The model under review builds one solid part; all positions refer to its coordinate system, in mm. Face numbers are marked on the shaded views. A direction names the side the tool comes from. Coordinates: 2 decimals unless noted, no trailing zeros. Loops run counter-clockwise (first coordinate to the right, second up) from the corner with the lowest first, then second, coordinate; pieces in that order, holes last. Notation, with made-up numbers: M 32.5,24.25 L 54.5,24.25 A14 ccw 54.5,51.25 Z; hole C 80.5,28 d5. An arc over 180 degrees is marked long. Use one line per item in the form item = value.
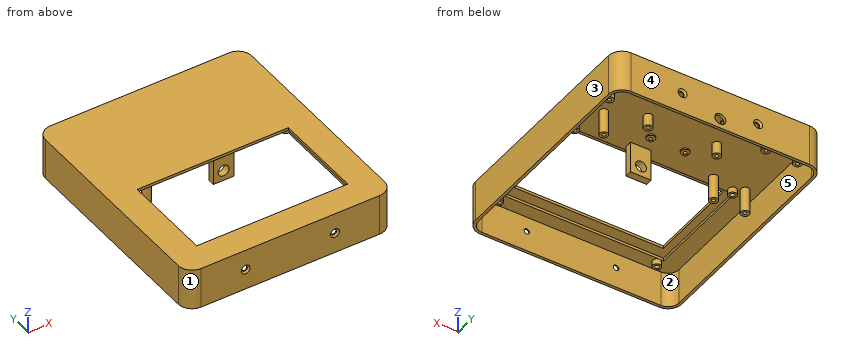
```python
from build123d import *

# Parameters (mm, degrees)
PAD_DEPTH           = 30
POCKET_DEPTH        = 26
SKETCH002_W         = 110
SKETCH002_H         = 66
POCKET001_DEPTH     = 5
SKETCH003_W         = 121
SKETCH003_H         = 78
POCKET002_DEPTH     = 2
SKETCH004_R         = 3
PAD001_DEPTH        = 4
SKETCH005_R         = 1.6
POCKET003_DEPTH     = 6
SKETCH006_R         = 3
PAD002_DEPTH        = 18
SKETCH007_R         = 1.3
POCKET004_DEPTH     = 8
SKETCH008_R         = 3
PAD003_DEPTH        = 1
SKETCH009_R         = 1
PAD004_DEPTH        = 2
SKETCH010_R         = 3
PAD005_DEPTH        = 9
SKETCH011_R         = 1.3
POCKET005_DEPTH     = 8
HOLE_D              = 4
HOLE_DEPTH          = 23.798279
HOLE_CSINK_D        = 6.5
HOLE_CSINK_ANGLE    = 90
HOLE_TIPS_R         = 2
HOLE001_D           = 4
HOLE001_DEPTH       = 23.798279
HOLE001_CSINK_D     = 6.5
HOLE001_CSINK_ANGLE = 90
HOLE001_TIPS_R      = 2
SKETCH014_R         = 4
POCKET006_DEPTH     = 5
SKETCH015_W         = 15
SKETCH015_H         = 5
PAD006_DEPTH        = 23
SKETCH016_R         = 4
POCKET007_DEPTH     = 5


with BuildPart() as part:
    # Sketch001 → Pad (new body)
    with BuildSketch(Plane.XY):
        with BuildLine():
            Line((10, 167), (140, 167))
            ThreePointArc((150, 157), (147.071068, 164.071068), (140, 167))
            Line((150, 157), (150, 10))
            ThreePointArc((140, 0), (147.071068, 2.928932), (150, 10))
            Line((140, 0), (10, 0))
            ThreePointArc((0, 10), (2.928932, 2.928932), (10, 0))
            Line((0, 10), (0, 157))
            ThreePointArc((10, 167), (2.928932, 164.071068), (0, 157))
        make_face()
    extrude(amount=PAD_DEPTH)

    # Sketch (on Face9 of Pad) → Pocket (cut)
    with BuildSketch(Plane(origin=(0, 0, 0), x_dir=(1, 0, 0), z_dir=(0, 0, -1))):
        with BuildLine():
            Line((9.999987, -2), (139.999987, -2))
            ThreePointArc((148, -10.000013), (145.65685, -4.34315), (139.999987, -2))
            Line((148, -10.000013), (148, -157.000013))
            ThreePointArc((140.000013, -165), (145.656858, -162.656858), (148, -157.000013))
            Line((140.000013, -165), (10.000013, -165))
            ThreePointArc((2, -156.999987), (4.34315, -162.65685), (10.000013, -165))
            Line((2, -156.999987), (2, -9.999987))
            ThreePointArc((9.999987, -2), (4.343142, -4.343142), (2, -9.999987))
        make_face()
    extrude(amount=-POCKET_DEPTH, mode=Mode.SUBTRACT)

    # Sketch002 (on Face19 of Pocket) → Pocket001 (cut)
    with BuildSketch(Plane(origin=(0, 0, 26), x_dir=(1, 0, 0), z_dir=(0, 0, -1))):
        with Locations((75, -53)):
            Rectangle(SKETCH002_W, SKETCH002_H)
    extrude(amount=-POCKET001_DEPTH, mode=Mode.SUBTRACT)

    # Sketch003 (on Face23 of Pocket001) → Pocket002 (cut)
    with BuildSketch(Plane(origin=(0, 0, 26), x_dir=(1, 0, 0), z_dir=(0, 0, -1))):
        with Locations((75, -51)):
            Rectangle(SKETCH003_W, SKETCH003_H)
    extrude(amount=-POCKET002_DEPTH, mode=Mode.SUBTRACT)

    # Sketch004 (on Face23 of Pocket002) → Pad001 (join)
    with BuildSketch(Plane(origin=(0, 0, 26), x_dir=(1, 0, 0), z_dir=(0, 0, -1))):
        with Locations((17.5, -9)):
            Circle(SKETCH004_R)
        with Locations((132.5, -9)):
            Circle(SKETCH004_R)
        with Locations((132.5, -93)):
            Circle(SKETCH004_R)
        with Locations((17.5, -93)):
            Circle(SKETCH004_R)
    extrude(amount=PAD001_DEPTH)

    # Sketch005 (on Face36 of Pad001) → Pocket003 (cut)
    with BuildSketch(Plane(origin=(0, 0, 22), x_dir=(1, 0, 0), z_dir=(0, 0, -1))):
        with Locations((17.5, -9)):
            Circle(SKETCH005_R)
        with Locations((132.5, -9)):
            Circle(SKETCH005_R)
        with Locations((17.5, -93)):
            Circle(SKETCH005_R)
        with Locations((132.5, -93)):
            Circle(SKETCH005_R)
    extrude(amount=-POCKET003_DEPTH, mode=Mode.SUBTRACT)

    # Sketch006 (on Face23 of Pocket003) → Pad002 (join)
    with BuildSketch(Plane(origin=(0, 0, 26), x_dir=(1, 0, 0), z_dir=(0, 0, -1))):
        with Locations((11, -97)):
            Circle(SKETCH006_R)
        with Locations((34, -97)):
            Circle(SKETCH006_R)
        with Locations((11, -155)):
            Circle(SKETCH006_R)
        with Locations((34, -155)):
            Circle(SKETCH006_R)
        with Locations((125, -114)):
            Circle(SKETCH006_R)
        with Locations((141, -144.565503)):
            Circle(SKETCH006_R)
    extrude(amount=PAD002_DEPTH)

    # Sketch007 (on Face39 of Pad002) → Pocket004 (cut)
    with BuildSketch(Plane(origin=(0, 0, 8), x_dir=(1, 0, 0), z_dir=(0, 0, -1))):
        with Locations((11, -97)):
            Circle(SKETCH007_R)
        with Locations((34, -97)):
            Circle(SKETCH007_R)
        with Locations((11, -155)):
            Circle(SKETCH007_R)
        with Locations((34, -155)):
            Circle(SKETCH007_R)
        with Locations((125, -114)):
            Circle(SKETCH007_R)
        with Locations((141, -144.565503)):
            Circle(SKETCH007_R)
    extrude(amount=-POCKET004_DEPTH, mode=Mode.SUBTRACT)

    # Sketch008 (on Face23 of Pocket004) → Pad003 (join)
    with BuildSketch(Plane(origin=(0, 0, 26), x_dir=(1, 0, 0), z_dir=(0, 0, -1))):
        with Locations((62.5, -109)):
            Circle(SKETCH008_R)
        with Locations((87.5, -109)):
            Circle(SKETCH008_R)
        with Locations((57.5, -146)):
            Circle(SKETCH008_R)
        with Locations((92.5, -146)):
            Circle(SKETCH008_R)
    extrude(amount=PAD003_DEPTH)

    # Sketch009 (on Face46 of Pad003) → Pad004 (join)
    with BuildSketch(Plane(origin=(0, 0, 25), x_dir=(1, 0, 0), z_dir=(0, 0, -1))):
        with Locations((62.5, -109)):
            Circle(SKETCH009_R)
        with Locations((92.5, -146)):
            Circle(SKETCH009_R)
        with Locations((87.5, -109)):
            Circle(SKETCH009_R)
        with Locations((57.5, -146)):
            Circle(SKETCH009_R)
    extrude(amount=PAD004_DEPTH)

    # Sketch010 (on Face23 of Pad004) → Pad005 (join)
    with BuildSketch(Plane(origin=(0, 0, 26), x_dir=(1, 0, 0), z_dir=(0, 0, -1))):
        with Locations((50, -125)):
            Circle(SKETCH010_R)
        with Locations((100, -125)):
            Circle(SKETCH010_R)
    extrude(amount=PAD005_DEPTH)

    # Sketch011 (on Face53 of Pad005) → Pocket005 (cut)
    with BuildSketch(Plane(origin=(0, 0, 17), x_dir=(1, 0, 0), z_dir=(0, 0, -1))):
        with Locations((100, -125)):
            Circle(SKETCH011_R)
        with Locations((50, -125)):
            Circle(SKETCH011_R)
    extrude(amount=-POCKET005_DEPTH, mode=Mode.SUBTRACT)

    # Hole
    with Locations(Plane(origin=(0, 167, 0), x_dir=(-1, 0, 0), z_dir=(0, 1, 0))):
        with Locations((-47.5, 15), (-102.5, 15)):
            CounterSinkHole(HOLE_D / 2, HOLE_CSINK_D / 2, depth=HOLE_DEPTH, counter_sink_angle=HOLE_CSINK_ANGLE)

    # Hole tips → Hole tip 1 section 0
    with BuildSketch(Plane(origin=(0, 143.201721, 0), x_dir=(-1, 0, 0), z_dir=(0, 1, 0)), mode=Mode.PRIVATE) as hole_tip_1_s0:
        with Locations((-47.5, 15)):
            Circle(HOLE_TIPS_R)
    loft([hole_tip_1_s0.sketch, Vertex(47.5, 142, 15)], mode=Mode.SUBTRACT)

    # Hole tips → Hole tip 2 section 0
    with BuildSketch(Plane(origin=(0, 143.201721, 0), x_dir=(-1, 0, 0), z_dir=(0, 1, 0)), mode=Mode.PRIVATE) as hole_tip_2_s0:
        with Locations((-102.5, 15)):
            Circle(HOLE_TIPS_R)
    loft([hole_tip_2_s0.sketch, Vertex(102.5, 142, 15)], mode=Mode.SUBTRACT)

    # Hole001
    with Locations(Plane.XZ):
        with Locations((42.5, 15), (107.5, 15)):
            CounterSinkHole(HOLE001_D / 2, HOLE001_CSINK_D / 2, depth=HOLE001_DEPTH, counter_sink_angle=HOLE001_CSINK_ANGLE)

    # Hole001 tips → Hole001 tip 1 section 0
    with BuildSketch(Plane.XZ.offset(-23.798279), mode=Mode.PRIVATE) as hole001_tip_1_s0:
        with Locations((42.5, 15)):
            Circle(HOLE001_TIPS_R)
    loft([hole001_tip_1_s0.sketch, Vertex(42.5, 25, 15)], mode=Mode.SUBTRACT)

    # Hole001 tips → Hole001 tip 2 section 0
    with BuildSketch(Plane.XZ.offset(-23.798279), mode=Mode.PRIVATE) as hole001_tip_2_s0:
        with Locations((107.5, 15)):
            Circle(HOLE001_TIPS_R)
    loft([hole001_tip_2_s0.sketch, Vertex(107.5, 25, 15)], mode=Mode.SUBTRACT)

    # Sketch014 (on Face7 of Hole001) → Pocket006 (cut)
    with BuildSketch(Plane(origin=(0, 167, 0), x_dir=(-1, 0, 0), z_dir=(0, 1, 0))):
        with Locations((-75, 7)):
            Circle(SKETCH014_R)
    extrude(amount=-POCKET006_DEPTH, mode=Mode.SUBTRACT)

    # Sketch015 (on Face28 of Pocket006) → Pad006 (join)
    with BuildSketch(Plane(origin=(0, 0, 26), x_dir=(1, 0, 0), z_dir=(0, 0, -1))):
        with Locations((87.5, -95.5)):
            Rectangle(SKETCH015_W, SKETCH015_H)
    extrude(amount=PAD006_DEPTH)

    # Sketch016 (on Face39 of Pad006) → Pocket007 (cut)
    with BuildSketch(Plane(origin=(0, 98, 0), x_dir=(-1, 0, 0), z_dir=(0, 1, 0))):
        with Locations((-87.5, 10.5)):
            Circle(SKETCH016_R)
    extrude(amount=-POCKET007_DEPTH, mode=Mode.SUBTRACT)


solid = part.part
```
1. Machinability: for the marked faces 4 and 5, which of the approach directions +Z, -Z, +X, -X, +Y, -Y give a long, thin tool a straight path to every point of the face, cutting with its end or side? Answer none if there is none.
Response values:
face_4 = +Z, -Z, +X, -X, +Y
face_5 = -Z
2. Add section A-A (y = 34). State the section outline as (x, z) points, then the cut area to 3 significant figures.
Response values:
outline = M 0,0 L 2,0 L 2,26 L 14.5,26 L 14.5,28 L 20,28 L 20,30 L 0,30 Z; M 130,28 L 135.5,28 L 135.5,26 L 148,26 L 148,0 L 150,0 L 150,30 L 130,30 Z
area = 242 mm^2
3. Insertion check: P1, Ø6.5, axis at x = 9.5, y = 96.5, coming from the -Z side; P2, Ø2, axis at x = 99.5, y = 125, coming from the -Z side; P3, Ø5, axis at x = 108, y = 85, coming from the -Z side. Each pin has a flat end and moves straight along its axis. Give the tip position at first contact, or say it passes through.
Response values:
P1 = 8
P2 = 17
P3 = 28
4. Wall thickness on line 1 along X through (y, z) = (155, 10.5); line 2 along Y through (x, z) = (17.5, 23.8); line 3 along X through (y, z) = (26.5, 7.5): over which ranges is each line inside the solid? List them lowest first. Write a range as from..to.
Response values:
line_1 = 0..2, 8..9.7, 12.3..14, 31..32.7, 35.3..37, 148..150
line_2 = 0..2, 6..7.4, 10.6..12, 90..91.4, 94.6..96, 165..167
line_3 = 0..2, 148..150
5. The part is to be moulded in two halves that separate along Y. For the marked faces 1, 2 and 3, say which applies: pulls with the +Y half, pulls with the -Y half, needs draft (parallel to the pull), parting line crosses it, or undercut.
Response values:
face_1 = pulls with the -Y half
face_2 = undercut
face_3 = needs draft
6. Add section B-B (x = 25.5). State the section outline as (y, z) points, then the cut area to 3 significant figures.
Response values:
outline = M 0,0 L 2,0 L 2,26 L 12,26 L 12,28 L 20,28 L 20,30 L 0,30 Z; M 86,28 L 90,28 L 90,26 L 165,26 L 165,0 L 167,0 L 167,30 L 86,30 Z
area = 484 mm^2
